```python
from build123d import *

# Parameters (mm, degrees)
SKETCH1_W           = 60
SKETCH1_H           = 50
BOSS_EXTRUDE1_DEPTH = 4
SKETCH2_W           = 60
SKETCH2_H           = 4
BOSS_EXTRUDE2_DEPTH = 4
FILLET1_R           = 4
BOSS_EXTRUDE3_DEPTH = 4
SKETCH3_R           = 2.25
CUT_EXTRUDE1_DEPTH  = 79.511145706


with BuildPart() as part:
    # Sketch1 → Boss-Extrude1 (new body)
    with BuildSketch(Plane.XY):
        with Locations((30, 25)):
            Rectangle(SKETCH1_W, SKETCH1_H)
    extrude(amount=BOSS_EXTRUDE1_DEPTH)

    # Sketch2 → Boss-Extrude2 (add)
    with BuildSketch(Plane(origin=(0, 0, 0), x_dir=(-1, 0, 0), z_dir=(0, 0, -1))):
        with Locations((-30, 19)):
            Rectangle(SKETCH2_W, SKETCH2_H)
    extrude(amount=BOSS_EXTRUDE2_DEPTH)

    # Fillet1
    fillet1_edges = [part.edges().sort_by_distance(p)[0] for p in [
        (30, 21, 0),
    ]]
    fillet(fillet1_edges, radius=FILLET1_R - 0.0001)  # a hair under: the kernel refuses the full size

    # Sketch6 → Boss-Extrude3 (add)
    with BuildSketch(Plane(origin=(0, 0, 0), x_dir=(-1, 0, 0), z_dir=(0, 0, -1))):
        with BuildLine():
            Line((0, 0), (0, 11))
            Line((0, 11), (-21, 11))
            ThreePointArc((-21, 11), (-25.242640687, 9.242640687), (-27, 5))
            Line((-27, 5), (-27, 0))
            Line((-27, 0), (0, 0))
        make_face()
        with BuildLine():
            Line((-33, 5), (-33, 0))
            Line((-33, 0), (-60, 0))
            Line((-60, 0), (-60, 11))
            Line((-60, 11), (-39, 11))
            ThreePointArc((-39, 11), (-34.757359313, 9.242640687), (-33, 5))
        make_face()
    extrude(amount=BOSS_EXTRUDE3_DEPTH)

    # Sketch3 → Cut-Extrude1 (cut, through all)
    with BuildSketch(Plane.XY.offset(4)):
        with Locations((12.5, 42.6)):
            Circle(SKETCH3_R)
        with Locations((55.5, 4.6)):
            Circle(SKETCH3_R)
    extrude(amount=-CUT_EXTRUDE1_DEPTH, mode=Mode.SUBTRACT)


solid = part.part
```
Source: CAD feature listing. Evaluate the final solid. Frame: model axes, mm. A direction names the side the tool comes from. Coordinates: 2 decimals unless noted, no trailing zeros. Loops run counter-clockwise (first coordinate to the right, second up) from the corner with the lowest first, then second, coordinate; pieces in that order, holes last. Notation, with made-up numbers: M 28,7.5 L 67,7.5 A10 cw 67,24.5 Z; hole C 17.25,48 d2. An arc over 180 degrees is marked long. Put each result on its own line as item: value. Start each with the question number.
1) Ray query, L1, parallel to Y at x = 12.5, z = 1.55; L2, parallel to Y at x = 55.5, z = -1.5; L3, parallel to X at y = 3, z = -0.75. Return the intervals inside material, ascending. Write a range as from..to.
2) Reachability of faces 4 (the face through (60, 19, 1)), 5 (the face through (46, 6, -4)), 6 (the face through (33, 3, -2)), 7 (the face through (30, 17, -2)), 8 (the face through (25.196, 9.289, -1.972)) from +Z, -Z, +X, -X, +Y, -Y: full face, straight path, thin tool, end or side. Return the list, or none.
3) Pull-direction query (Y, two-part tool) for faces 1 (the face through (14, 6, -4)), 2 (the face through (30, 50, 2)), 3 (the face through (10, 11, -2)); classes: pulls with the +Y half, pulls with the -Y half, needs draft (parallel to the pull), parting line crosses it, or undercut.
4) Cut plane C-C on z = -1. Return the cut outline in (x, y), then the cut area to 3 significant figures.
5) Contact query for flat-ended pins moving along their axis: pin 1 Ø3 at (x, z) = (54, -2.5) entering from +Y; pin 2 Ø8 at (x, y) = (6.5, 39) entering from -Z; pin 3 Ø1.5 at (y, z) = (24.5, -1) entering from +X. Output: stop coordinate, or through.
6) Cut plane B-B on y = 42.6. Return the cut outline in (x, z), then the cut area to 3 significant figures.
The answers:
1. L1: y = 0..40.35, 44.85..50
1. L2: y = 0..2.35, 6.85..11, 17..21.88
1. L3: x = 0..27, 33..53.92, 57.08..60
2. face 4: +Z, -Z, +X, +Y, -Y
2. face 5: -Z, +X, -X, +Y, -Y
2. face 6: -Z, -Y
2. face 7: -Z, +X, -X
2. face 8: -Z
3. face 1: needs draft
3. face 2: pulls with the +Y half
3. face 3: undercut
4. outline: M 0,0 L 27,0 L 27,5 A6 ccw 21,11 L 0,11 Z; M 0,17 L 60,17 L 60,22.35 L 0,22.35 Z; M 33,0 L 60,0 L 60,11 L 39,11 A6 ccw 33,5 Z; hole C 55.5,4.6 d4.5
4. area: 884 mm²
5. pin 1: stops at y = 22.35
5. pin 2: stops at z = 0
5. pin 3: passes through
6. outline: M 0,0 L 10.25,0 L 10.25,4 L 0,4 Z; M 14.75,0 L 60,0 L 60,4 L 14.75,4 Z
6. area: 222 mm²
